Read the model definition and answer for the solid it produces. Units are mm, in the model's axes. Face numbers are marked on the shaded views. A direction names the side the tool comes from. Give positions to 0.01 mm unless a question says otherwise; leave off trailing zeros. Write each loop counter-clockwise with the first axis right and the second up, starting at its lowest first coordinate (ties: lowest second). Pieces come first, ordered by that corner, then holes. Notation, with made-up numbers: M 68,11.25 L 74,11.25 A10 ccw 74,25.25 Z; hole C -25.75,63 d8. An arc over 180 degrees is marked long. Write each question's results on one line, items separated by ' | '. Start each with the question number.
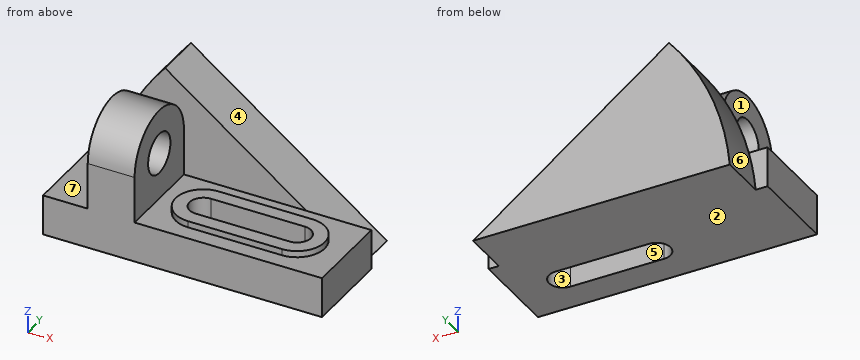
```python
from build123d import *

# Parameters (mm, degrees)
F0_W      = 131
F0_H      = 19
F1_DEPTH  = 42
F2_W      = 22
F2_H      = 22
F3_DEPTH  = 42
F5_DEPTH  = 22
F6_R      = 9.5
F7_DEPTH  = 43.001
F9_DEPTH  = 19.001
F12_DEPTH = 22
F13_DEPTH = 3


with BuildPart() as f1:
    # F0 (on Front) → F1 (new body)
    with BuildSketch(Plane.XZ):
        with Locations((65.5, 9.5)):
            Rectangle(F0_W, F0_H)
    extrude(amount=-F1_DEPTH)

    # F2 (on face) → F3 (join)
    with BuildSketch(Plane.XZ):
        with Locations((32, 30)):
            Rectangle(F2_W, F2_H)
    extrude(amount=-F3_DEPTH)

    # F4 (on face) → F5 (join)
    with BuildSketch(Plane.YZ.offset(43)):
        with BuildLine():
            Line((0, 41), (42, 41))
            ThreePointArc((42, 41), (21, 62), (0, 41))
        make_face()
    extrude(amount=-F5_DEPTH)

    # F6 (on face) → F7 (cut, through all)
    with BuildSketch(Plane.YZ.offset(43)):
        with Locations((21, 41)):
            Circle(F6_R)
    extrude(amount=-F7_DEPTH, mode=Mode.SUBTRACT)

    # F8 (on face) → F9 (cut, through all)
    with BuildSketch(Plane.XY.offset(19)):
        with BuildLine():
            ThreePointArc((64, 27), (57.5, 20.5), (64, 14))
            Line((64, 14), (108, 14))
            ThreePointArc((108, 14), (114.5, 20.5), (108, 27))
            Line((108, 27), (64, 27))
        make_face()
    extrude(amount=-F9_DEPTH, mode=Mode.SUBTRACT)

    # F11 (on face) → F12 (join)
    with BuildSketch(Plane(origin=(0, 42, 0), x_dir=(-1, 0, 0), z_dir=(0, 1, 0))):
        with BuildLine():
            Line((-34.1583360178, 68.1544452659), (-126.1935941596, 0))
            Line((-126.1935941596, 0), (-5.6412019979, 0))
            ThreePointArc((-5.6412019979, 0), (-14.5708616504, 36.3069402207), (-34.1583360178, 68.1544452659))
        make_face()
    extrude(amount=F12_DEPTH)

    # F10 (on face) → F13 (join)
    with BuildSketch(Plane.XY.offset(19)):
        with BuildLine():
            Line((108, 33.4034413099), (64, 33.4034413099))
            ThreePointArc((64, 33.4034413099), (51, 20.4034413099), (64, 7.4034413099))
            Line((64, 7.4034413099), (108, 7.4034413099))
            ThreePointArc((108, 7.4034413099), (121, 20.4034413099), (108, 33.4034413099))
        make_face()
        with BuildLine():
            Line((108, 14), (64, 14))
            ThreePointArc((64, 14), (57.5, 20.5), (64, 27))
            Line((64, 27), (108, 27))
            ThreePointArc((108, 27), (114.5, 20.5), (108, 14))
        make_face(mode=Mode.SUBTRACT)
    extrude(amount=F13_DEPTH)


solid = f1.part
```
Item 1: Straight lines are drawn through the part: line 1 (Y direction, x = 66.5, z = 21); line 2 (Z direction, x = 27, y = 21); line 3 (Y direction, x = 107.5, z = 8). For each, find the intervals that lie inside material, in ascending order.
Item 2: Given P1, Ø12.5, axis at y = 19, z = 33.5, coming from the +X side; P2, Ø8, axis at x = 78.5, y = 24, coming from the +Z side; P3, Ø1, axis at x = 46, y = 20, coming from the +Z side, each flat-ended and moving along its own axis, determine where each tip first touches the part or whether it passes through.
Item 3: Section D-D, the plane z = 17.5 is taken. Determine the outline of the cut face in (x, y), then the cut area to 3 significant figures.
Item 4: For the marked faces 4, 5, 6 and 7, determine the directions among +Z, -Z, +X, -X, +Y, -Y from which every point of the face is accessible in a straight line to the end or side of a thin tool.
Item 5: Section A-A, the plane z = 37.5 is taken. Determine the outline of the cut face in (x, y), then the cut area to 3 significant figures.
Item 6: Section C-C, the plane x = 95.5 is taken. Determine the outline of the cut face in (y, z), then the cut area to 3 significant figures.
Item 7: Determine the mould class of the marked faces 1, 2 and 3 for opening direction X: +X half, -X half, draft (parallel to the pull), parting line (faces both ways), or undercut.
Item 8: Section B-B, the plane y = 23 is taken. Determine the outline of the cut face in (x, z).
Worked out:
1) line 1: y = 7.4 to 14, 27 to 33.4, 42 to 64 | line 2: z = 0 to 31.5, 50.5 to 62 | line 3: y = 0 to 14, 27 to 64
2) P1: stops at x = 43 | P2: stops at z = 22 | P3: stops at z = 19
3) outline: M 0,0 L 131,0 L 131,42 L 102.56,42 L 102.56,64 L 8.45,64 L 8.45,42 L 0,42 Z; hole M 64,14 L 108,14 A6.5 ccw 108,27 L 64,27 A6.5 ccw Z | area: 6,870 mm²
4) face 4: +Z, +X, +Y | face 5: +Z, -Z | face 6: +Z, -X, +Y | face 7: +Z, -X, -Y
5) outline: M 15.08,42 L 21,42 L 21,29.83 L 43,29.83 L 43,42 L 75.55,42 L 75.55,64 L 15.08,64 Z; M 21,0 L 43,0 L 43,12.17 L 21,12.17 Z | area: 1,870 mm²
6) outline: M 0,0 L 14,0 L 14,22 L 7.4,22 L 7.4,19 L 0,19 Z; M 27,0 L 64,0 L 64,22.73 L 42,22.73 L 42,19 L 33.4,19 L 33.4,22 L 27,22 Z | area: 1,090 mm²
7) face 1: -X half | face 2: draft | face 3: undercut
8) outline: M 0,0 L 58,0 L 58,22 L 51.26,22 L 51.26,19 L 43,19 L 43,31.71 L 21,31.71 L 21,19 L 0,19 Z; M 21,50.29 L 43,50.29 L 43,61.9 L 21,61.9 Z; M 114,0 L 131,0 L 131,19 L 120.74,19 L 120.74,22 L 114,22 Z
